Autodesk Inventor part; units mm, degrees
sketch "Esboço1" plane through (0, 0, 0) normal (0, 0, 1) x (1, 0, 0)
  line L0 (-15, -15) -> (15, -15)
  line L1 (15, -15) -> (15, 15)
  line L2 (15, 15) -> (-15, 15)
  line L3 (-15, 15) -> (-15, -15)
  line L4 (-15, -15) -> (15, 15) construction
  line L5 (15, -15) -> (-15, 15) construction
  circle A0 centre (0, 10.49) radius 2.51
  point P0 (0, 0)
  dimension "d0" = 30
  dimension "d4" = 5.02
  dimension "d5" = 2
extrude "Extrusão1" add sketch "Esboço1" along normal mid plane 10
fillet "Arredondamento1" radius 3 4 edges at (-15, 15, 0) (15, 15, 0) (15, -15, 0) (-15, -15, 0)
chamfer "Chanfro1" distance 1 angle 45 1 edges at (-2.51, 10.49, 5)
properties part number "Sessao8_07_04_2025_0004_0001" material "Ouro"
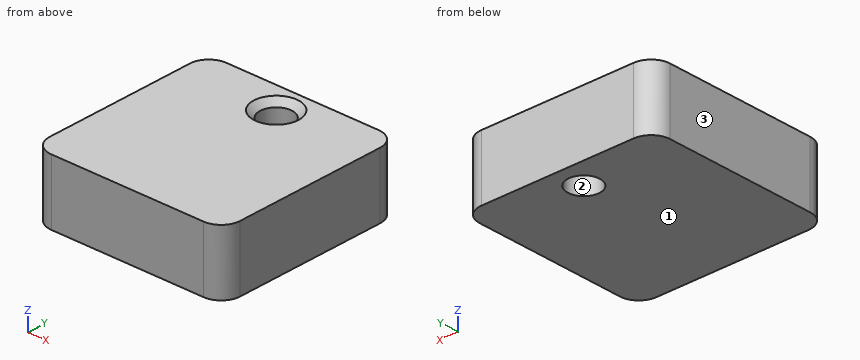
For this review, take the finished solid that the model builds, in its own axes (mm). Face numbers are marked on the shaded views. Round coordinates to 2 decimals unless told otherwise and drop trailing zeros. Loops run counter-clockwise (first coordinate to the right, second up) from the corner with the lowest first, then second, coordinate; pieces in that order, holes last.
Q1. Add section C-C on z = 3.25. Write out the cut boundary in (x, y), plus the area to 3 significant figures.
Result sheet:
outline: (-15, -12) arc R3 ccw to (-12, -15) - (12, -15) arc R3 ccw to (15, -12) - (15, 12) arc R3 ccw to (12, 15) - (-12, 15) arc R3 ccw to (-15, 12) - close; hole circle Ø5.02 at (0, 10.49)
area: 872 mm2
Q2. Add section A-A on y = 10.49. Write out the cut boundary in (x, z), plus the area to 3 significant figures.
Result sheet:
outline: (-15, -5) - (-2.51, -5) - (-2.51, 4) - (-3.51, 5) - (-15, 5) - close; (2.51, -5) - (15, -5) - (15, 5) - (3.51, 5) - (2.51, 4) - close
area: 249 mm2
Q3. Add section B-B on x = 0. Write out the cut boundary in (y, z).
Result sheet:
outline: (-15, -5) - (7.98, -5) - (7.98, 4) - (6.98, 5) - (-15, 5) - close; (13, -5) - (15, -5) - (15, 5) - (14, 5) - (13, 4) - close
Q4. Mouldability with a two-part tool opening along X and no side actions: class the marked faces 1, 2 and 3 as +X half, -X half, draft (parallel to the pull), parting line (faces both ways), or undercut.
Result sheet:
face 1: draft
face 2: undercut
face 3: -X half
Q5. To check wall thickness, follow line 1 along Y through (x, z) = (0, 0); line 2 along X through (y, z) = (10, 3.75); line 3 along X through (y, z) = (12, 2.25) (3 decimals). State the ranges of each line that lie inside material, in increasing order.
Result sheet:
line 1: y = -15 to 7.98, 13 to 15
line 2: x = -15 to -2.46, 2.46 to 15
line 3: x = -15 to -2.005, 2.005 to 15
Q6. Insertion check: pin 1 Ø3 at (x, y) = (0, 10.49) entering from -Z. The pin has a flat end and moves straight along its axis. Give the tip position at first contact, or say it passes through.
Result sheet:
pin 1: passes through
